```python
from build123d import *

# Parameters (mm, degrees)
MAIN_EXTRUDE_DEPTH        = 101.6
MOUNTING_HOLES_D          = 5.1054
MOUNTING_HOLES_DEPTH      = 16.51
MOUNTING_HOLES_TIP        = 1.533816902
BEARING_MOUNT_LEFT_D      = 5.1054
BEARING_MOUNT_LEFT_DEPTH  = 12.7
BEARING_MOUNT_LEFT_TIP    = 1.533816902
BEARING_MOUNT_RIGHT_D     = 5.1054
BEARING_MOUNT_RIGHT_DEPTH = 16.51
BEARING_MOUNT_RIGHT_TIP   = 1.533816902


with BuildPart() as part:
    # Sketch2 → Main extrude (new body)
    with BuildSketch(Plane.XY):
        Polygon((-91.469223626, 25.4), (-53.369223626, -12.7), (-15.269223626, 25.4), align=None)
    extrude(amount=MAIN_EXTRUDE_DEPTH)

    # Mounting holes
    with Locations(Plane(origin=(0, 25.4, 0), x_dir=(1, 0, 0), z_dir=(0, 1, 0))):
        with Locations((-53.369223626, -19.05), (-53.369223626, -82.55), (-53.369223626, -50.8)):
            Hole(MOUNTING_HOLES_D / 2, depth=MOUNTING_HOLES_DEPTH)
            with Locations((0, 0, -(MOUNTING_HOLES_DEPTH + MOUNTING_HOLES_TIP / 2))):  # 118° drill point
                Cone(0, MOUNTING_HOLES_D / 2, MOUNTING_HOLES_TIP, mode=Mode.SUBTRACT)

    # Bearing mount left
    with Locations(Plane(origin=(-20.334611813, 20.334611813, 0), x_dir=(-0.707106781, -0.707106781, 0), z_dir=(0.707106781, -0.707106781, 0))):
        with Locations((21.317996054, -12.7), (21.317996054, -88.9)):
            Hole(BEARING_MOUNT_LEFT_D / 2, depth=BEARING_MOUNT_LEFT_DEPTH)
            with Locations((0, 0, -(BEARING_MOUNT_LEFT_DEPTH + BEARING_MOUNT_LEFT_TIP / 2))):  # 118° drill point
                Cone(0, BEARING_MOUNT_LEFT_D / 2, BEARING_MOUNT_LEFT_TIP, mode=Mode.SUBTRACT)

    # Bearing mount right
    with Locations(Plane(origin=(-33.034611813, -33.034611813, 0), x_dir=(-0.707106781, 0.707106781, 0), z_dir=(-0.707106781, -0.707106781, 0))):
        with Locations((54.157483812, -82.55), (54.157483812, -19.05)):
            Hole(BEARING_MOUNT_RIGHT_D / 2, depth=BEARING_MOUNT_RIGHT_DEPTH)
            with Locations((0, 0, -(BEARING_MOUNT_RIGHT_DEPTH + BEARING_MOUNT_RIGHT_TIP / 2))):  # 118° drill point
                Cone(0, BEARING_MOUNT_RIGHT_D / 2, BEARING_MOUNT_RIGHT_TIP, mode=Mode.SUBTRACT)


solid = part.part
```
Here's how the part is built. I have some questions about the finished solid (model axes, mm). A direction names the side the tool comes from. Round coordinates to 2 decimals unless told otherwise and drop trailing zeros. Write each loop counter-clockwise with the first axis right and the second up, starting at its lowest first coordinate (ties: lowest second). Pieces come first, ordered by that corner, then holes.
Q1. Will these pins go through, and if not, where does the flat tip stop? P1, Ø1.5, axis at x = -25.5, y = 12, coming from the +Z side (3 decimals); P2, Ø10, axis at y = -5, z = 62.5, coming from the +X side; P3, Ø4.5, axis at x = -53.37, z = 82.55, coming from the -Y side; P4, Ø2, axis at x = -42, z = 87, coming from the -Y side.
Q2. If we section it at C-C on y = 14: Give the number of separate pieces and of enclosed holes in the cut face, plus the area to 3 significant figures.
Q3. If we section it at B-B on z = 39: Write out the boundary of the cut face in (x, y), plus the area to 3 significant figures.
Q4. Please list where these lines run through material, in increasing order: probe 1 along Z at (x, y) = (-39, 8.5); probe 2 along Z at (x, y) = (-63, 17); probe 3 along X at (y, z) = (18, 50.8).
Q5. If we section it at A-A on y = 21.5: Write out the boundary of the cut face in (x, z), plus the area to 3 significant figures.
Q6. If we mould it in two halves opening along Z, with no side actions, what happens to faces 4 (the flat face through (-72.69, 6.62, 50.09)), 5 (the flat face through (-54, 11, 0)), 6 (the flat face through (-54, 11, 101.6)), 7 (the cylindrical face through (-55.804, 17.029, 18.283))? For each: +Z half, -Z half, draft (parallel to the pull), parting line (faces both ways), or undercut.
Q7. Which directions (+Z, -Z, +X, -X, +Y, -Y) give clear straight access to the entire face, cutting with the end or side of a thin tool? Please do faces 1 (the flat face through (-34.59, 6.08, 50.09)), 2 (the cylindrical face through (-55.804, 17.029, 81.783)), 3 (the conical face through (-58.9, 18, 18.7)).
Answer below:
1. P1: passes through
1. P2: stops at x = -40.67
1. P3: stops at y = -12.7
1. P4: stops at y = -2.33
2. separate pieces: 1
2. enclosed holes: 7
2. area: 5,260 mm2
3. outline: (-91.47, 25.4) - (-53.37, -12.7) - (-15.27, 25.4) - close
3. area: 1,450 mm2
4. probe 1: z = 0 to 10.16, 15.24 to 86.36, 91.44 to 101.6
4. probe 2: z = 0 to 18.21, 19.89 to 81.71, 83.39 to 101.6
4. probe 3: x = -84.07 to -55.92, -50.82 to -22.67
5. outline: (-87.57, 0) - (-19.17, 0) - (-19.17, 101.6) - (-87.57, 101.6) - close; hole circle Ø5.11 at (-53.37, 19.05); hole circle Ø5.11 at (-53.37, 50.8); hole circle Ø5.11 at (-53.37, 82.55)
5. area: 6,890 mm2
6. face 4: draft
6. face 5: -Z half
6. face 6: +Z half
6. face 7: undercut
7. face 1: +Z, -Z, +X, -Y
7. face 2: +Y
7. face 3: none
